Can you work these out from the drawing? Everything is in mm from the part's minimum corner. Round coordinates to 2 decimals unless told otherwise and drop trailing zeros. Write each loop counter-clockwise with the first axis right and the second up, starting at its lowest first coordinate (ties: lowest second). Pieces come first, ordered by that corner, then holes. Notation, with made-up numbers: M 24,18.25 L 67,18.25 A23 cw 67,45.25 Z; hole C 72,40 d6. An arc over 180 degrees is marked long. Answer in a Markdown table with one row per item. Add a question column.
(1) Suppose I cut it at A-A, the plane y = 175.5. Write out the boundary of the cut face in (x, z), then the cut area to 3 significant figures.
(2) I'm going to push flat-ended pins straight in: pin 1 (1 mm diameter, centred on x = 51, z = 1.5, fed in from -Y); pin 2 (6.5 mm diameter, centred on x = 126, z = 5, fed in from -Y) (1 decimal). Where does each tip first touch, or does it pass through?
(3) Suppose I cut it at D-D, the plane y = 95. Write out the boundary of the cut face in (x, z) (1 decimal).
(4) Suppose I cut it at C-C, the plane x = 116. Write out the boundary of the cut face in (y, z) (1 decimal).
(5) If I drill on probe 1 along X at (y, z) = (102, 6.25) (1 decimal); probe 2 along X at (y, z) = (37, 1) (1 decimal); probe 3 along X at (y, z) = (191, 4.75) (1 decimal), over which ranges is the centre line in solid material (lowest first)?
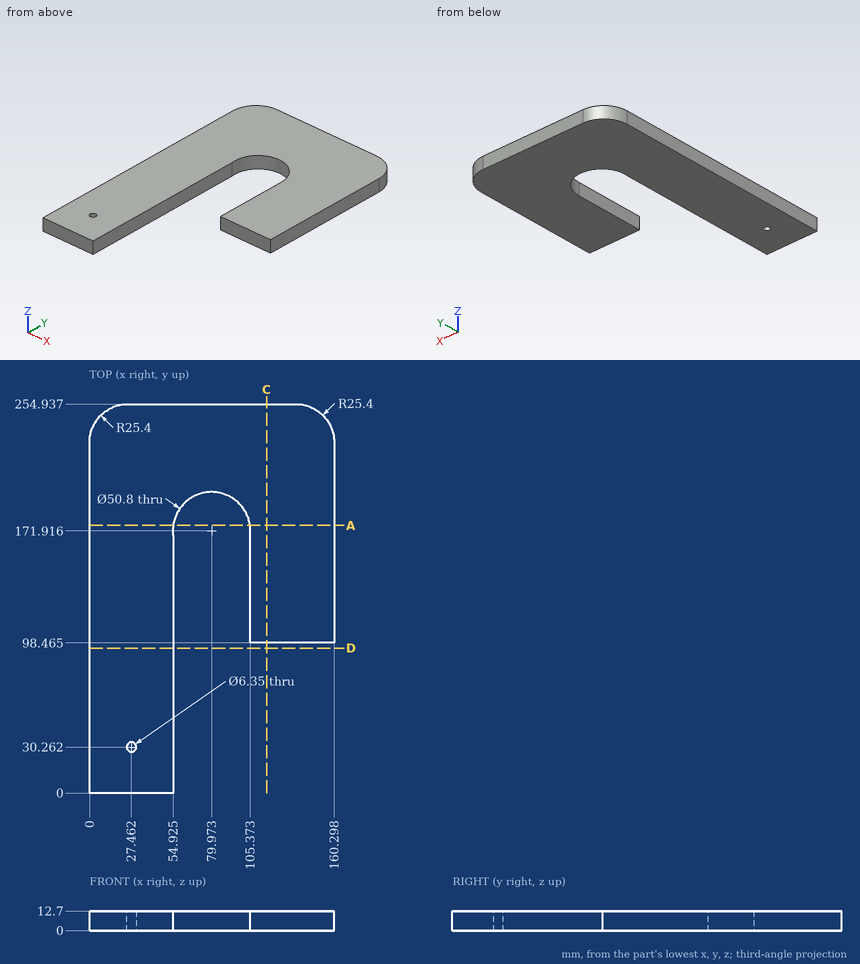
Calculated:
| question | item | result |
|---|---|---|
| 1 | outline | M 0,0 L 54.83,0 L 54.83,12.7 L 0,12.7 Z; M 105.12,0 L 160.3,0 L 160.3,12.7 L 105.12,12.7 Z |
| 1 | area | 1,400 mm² |
| 2 | pin 1 | y = 0 |
| 2 | pin 2 | y = 98.5 |
| 3 | outline | M 0,0 L 54.9,0 L 54.9,12.7 L 0,12.7 Z |
| 4 | outline | M 98.5,0 L 254.9,0 L 254.9,12.7 L 98.5,12.7 Z |
| 5 | probe 1 | 0 to 54.9, 105.4 to 160.3 |
| 5 | probe 2 | 0 to 54.9 |
| 5 | probe 3 | 0 to 63.2, 96.7 to 160.3 |
